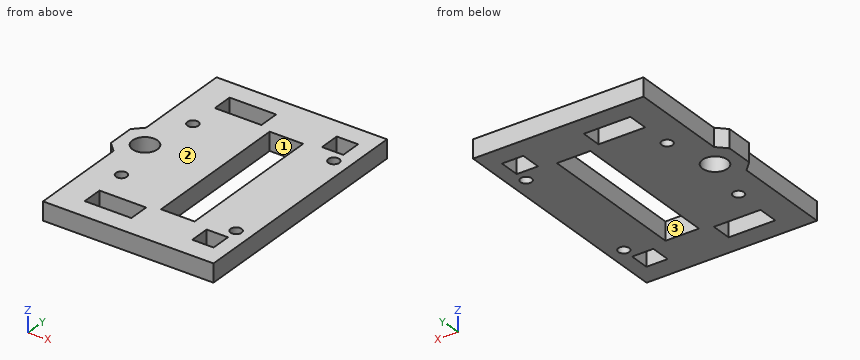
from build123d import *

# Parameters (mm, degrees)
MODEL_R                  = 1.8
MODEL_R_2                = 4.1
MODEL_W                  = 10.999995004
MODEL_H                  = 49.999979697
MODEL_W_2                = 7
MODEL_H_2                = 6.6
MODEL_W_3                = 15.312275424
MODEL_H_3                = 6.8
RESSALTO_EXTRUS_O1_DEPTH = 6


with BuildPart() as part:
    # Model → Ressalto-extrusão1 (new body)
    with BuildSketch(Plane.XY):
        Polygon((30.677261567, 6.624591957), (30.677261567, 39.085505862), (27.677261567, 42.085505862), (27.677261567, 51.063678051), (30.677261567, 54.063678051), (30.677261567, 86.524591957), (86.677261567, 86.524591957), (86.677261567, 6.624591957), align=None)
        with Locations((81.677261567, 24.074591957)):
            Circle(MODEL_R, mode=Mode.SUBTRACT)
        with Locations((39.677261567, 30.124591957)):
            Circle(MODEL_R, mode=Mode.SUBTRACT)
        with Locations((35.677261567, 46.574591957)):
            Circle(MODEL_R_2, mode=Mode.SUBTRACT)
        with Locations((39.677261567, 63.024591957)):
            Circle(MODEL_R, mode=Mode.SUBTRACT)
        with Locations((81.677261567, 69.074591957)):
            Circle(MODEL_R, mode=Mode.SUBTRACT)
        with Locations((64.294725156, 46.574591957)):
            Rectangle(MODEL_W, MODEL_H, mode=Mode.SUBTRACT)
        with Locations((78.377261567, 16.724591957)):
            Rectangle(MODEL_W_2, MODEL_H_2, mode=Mode.SUBTRACT)
        with Locations((47.333399279, 16.624591957)):
            Rectangle(MODEL_W_3, MODEL_H_3, mode=Mode.SUBTRACT)
        with Locations((47.333399279, 76.524591957)):
            Rectangle(MODEL_W_3, MODEL_H_3, mode=Mode.SUBTRACT)
        with Locations((78.377261567, 76.524591957)):
            Rectangle(MODEL_W_2, MODEL_H_3, mode=Mode.SUBTRACT)
    extrude(amount=RESSALTO_EXTRUS_O1_DEPTH)


solid = part.part
Source: CAD feature listing. Evaluate the final solid. Frame: model axes, mm. Face numbers are marked on the shaded views. Give positions to 0.01 mm unless a question says otherwise; leave off trailing zeros. Write each loop counter-clockwise with the first axis right and the second up, starting at its lowest first coordinate (ties: lowest second). Pieces come first, ordered by that corner, then holes. Notation, with made-up numbers: (3, -16.75) -> (12, -16.75) arc R21 cw to (12, -0.75) -> close; hole circle Ø10 at (-9.75, -34.75). An arc over 180 degrees is marked (long way). Return JSON: item names as keys, results as strings. Group by question number.
1. Material intervals for line 1 (Y direction, x = 75.5, z = 0.75); line 2 (Y direction, x = 54, z = 4.95); line 3 (X direction, y = 69, z = 5.2), sorted ascending. Write a range as from..to.
2. Pin query (flat end, axial travel): pin 1 Ø3 at (y, z) = (76, 3) entering from -X; pin 2 Ø3 at (y, z) = (40, 4) entering from -X; pin 3 Ø3 at (y, z) = (41, 3) entering from -X. Return the tip coordinate at first contact, or that it passes through.
3. Section B-B, the plane x = 78. Output: boundary loops of the cut face in (y, z), then the cut area to 3 significant figures.
4. Section A-A, the plane y = 74.5. Output: boundary loops of the cut face in (x, z).
5. Section C-C, the plane x = 67. Output: boundary loops of the cut face in (y, z).
6. Mould query, pull axis X, two halves, no side actions, for the marked faces 1, 2 and 3. Classes: +X half, -X half, draft (parallel to the pull), parting line (faces both ways), or undercut.
7. Section D-D, the plane z = 3.25. Count the separate pieces of the cut face and the enclosed holes in it, then the cut area to 3 significant figures.
Determined:
{
 "1": {"line 1": "y = 6.62..13.42, 20.02..73.12, 79.92..86.52", "line 2": "y = 6.62..13.22, 20.02..73.12, 79.92..86.52", "line 3": "x = 30.68..58.79, 69.79..79.88, 83.48..86.68"},
 "2": {"pin 1": "stops at x = 30.68", "pin 2": "stops at x = 28.26", "pin 3": "stops at x = 27.68"},
 "3": {"outline": "(6.62, 0) -> (13.42, 0) -> (13.42, 6) -> (6.62, 6) -> close; (20.02, 0) -> (73.12, 0) -> (73.12, 6) -> (20.02, 6) -> close; (79.92, 0) -> (86.52, 0) -> (86.52, 6) -> (79.92, 6) -> close", "area": "399 mm2"},
 "4": {"outline": "(30.68, 0) -> (39.68, 0) -> (39.68, 6) -> (30.68, 6) -> close; (54.99, 0) -> (74.88, 0) -> (74.88, 6) -> (54.99, 6) -> close; (81.88, 0) -> (86.68, 0) -> (86.68, 6) -> (81.88, 6) -> close"},
 "5": {"outline": "(6.62, 0) -> (21.57, 0) -> (21.57, 6) -> (6.62, 6) -> close; (71.57, 0) -> (86.52, 0) -> (86.52, 6) -> (71.57, 6) -> close"},
 "6": {"face 1": "undercut", "face 2": "draft", "face 3": "undercut"},
 "7": {"separate pieces": "1", "enclosed holes": "10", "area": "3,560 mm2"}
}
